For this review, use the dimensioned drawing (mm, ordinates from the lowest corner) and the shaded views. Give positions to 0.01 mm unless a question says otherwise; leave off trailing zeros. Write each loop counter-clockwise with the first axis right and the second up, starting at its lowest first coordinate (ties: lowest second). Pieces come first, ordered by that corner, then holes. Notation, with made-up numbers: M 21.25,45 L 64.25,45 A30 cw 64.25,81 Z; hole C -34.75,16.5 d6. An arc over 180 degrees is marked long. One line per item, written item: value. Start each with the question number.
Item 1: Consider section C-C, the plane x = 0.55. Write out the cut boundary in (y, z).
Item 2: Consider section A-A, the plane z = 1.25. Write out the cut boundary in (x, y), and give its area (3 significant figures).
Item 3: Consider section B-B, the plane y = 4.5. Write out the cut boundary in (x, z), and give its area (3 significant figures).
Item 4: Consider section D-D, the plane z = 1.7. Write out the cut boundary in (x, y).
Item 5: Clearance check with flat-ended pins moving along their axes: pin 1 Ø0.7 at (y, z) = (1.5, 1) entering from +X; pin 2 Ø0.5 at (x, y) = (1.5, 1.5) entering from -Z; pin 3 Ø0.7 at (x, y) = (1.5, 2) entering from +Z. State where each tip first meets the part, or that it passes through.
Item 6: To check wall thickness, follow probe 1 along Y at (x, z) = (1.15, 0.4); probe 2 along X at (y, z) = (9.75, 1.35). State the ranges of each line that lie inside material, in increasing order.
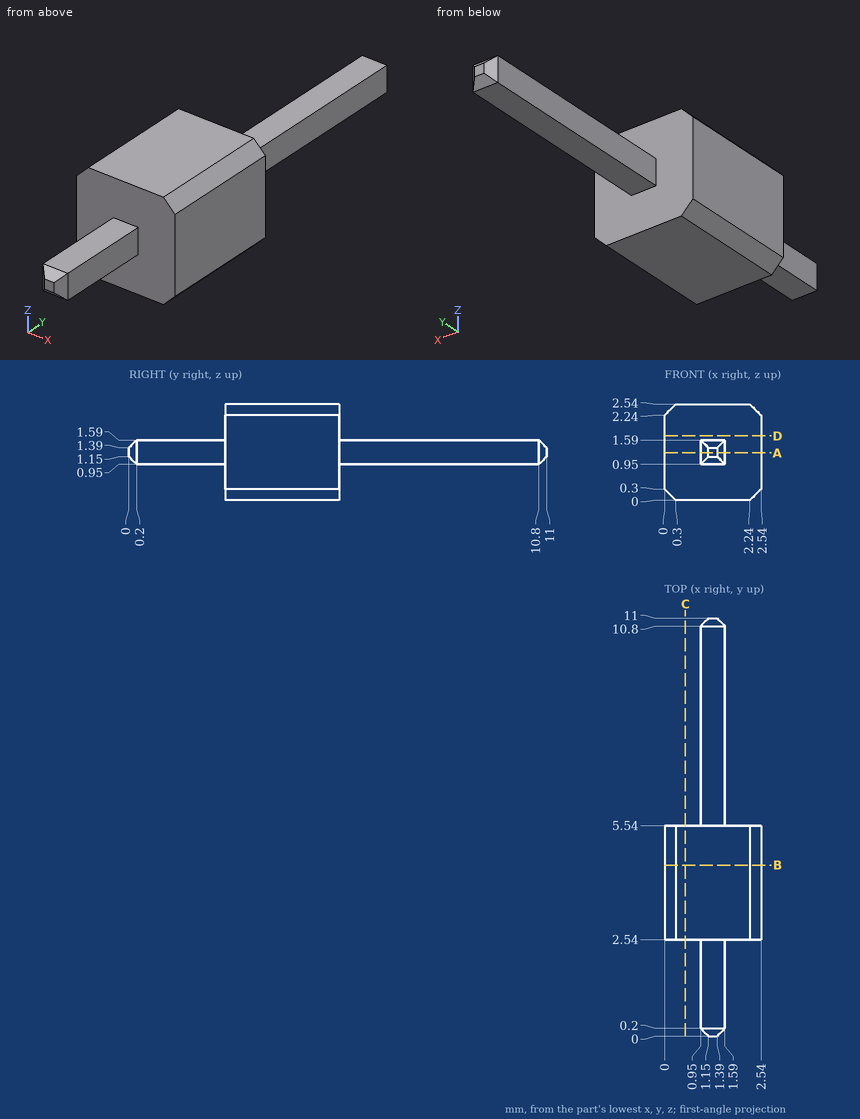
Model answer:
1. outline: M 2.54,0 L 5.54,0 L 5.54,2.54 L 2.54,2.54 Z
2. outline: M 0,2.54 L 0.95,2.54 L 0.95,0.2 L 1.15,0 L 1.39,0 L 1.59,0.2 L 1.59,2.54 L 2.54,2.54 L 2.54,5.54 L 1.59,5.54 L 1.59,10.8 L 1.39,11 L 1.15,11 L 0.95,10.8 L 0.95,5.54 L 0,5.54 Z
2. area: 12.7 mm2
3. outline: M 0,0.3 L 0.3,0 L 2.24,0 L 2.54,0.3 L 2.54,2.24 L 2.24,2.54 L 0.3,2.54 L 0,2.24 Z
3. area: 6.27 mm2
4. outline: M 0,2.54 L 2.54,2.54 L 2.54,5.54 L 0,5.54 Z
5. pin 1: stops at x = 1.59
5. pin 2: stops at z = 0.95
5. pin 3: stops at z = 1.59
6. probe 1: y = 2.54 to 5.54
6. probe 2: x = 0.95 to 1.59
